from build123d import *

# Parameters (mm, degrees)
SKETCH1_R           = 2.2
BOSS_EXTRUDE1_DEPTH = 22.2504
FILLET1_R           = 10
FILLET2_R           = 2
FILLET3_R           = 4
FILLET4_R           = 1.5
SKETCH2_R           = 2.15
CUT_EXTRUDE1_DEPTH  = 88.351467531


with BuildPart() as part:
    # Sketch1 → Boss-Extrude1 (new body)
    with BuildSketch(Plane(origin=(0, 0, 0), x_dir=(1, 0, 0), z_dir=(0, 1, 0))):
        Polygon((-5, 6.0452), (28.7, 6.0452), (28.7, 57.4548), (-5, 57.4548), (-5, 69.5452), (37.7, 69.5452), (37.7, -6.0452), (-5, -6.0452), align=None)
        with Locations(Location((0, 0, 0), (0, 0, 90))):
            Circle(SKETCH1_R, mode=Mode.SUBTRACT)
        with Locations(Location((12.7, 0, 0), (0, 0, 90))):
            Circle(SKETCH1_R, mode=Mode.SUBTRACT)
        with Locations(Location((12.7, 63.5, 0), (0, 0, 90))):
            Circle(SKETCH1_R, mode=Mode.SUBTRACT)
        with Locations(Location((0, 63.5, 0), (0, 0, 90))):
            Circle(SKETCH1_R, mode=Mode.SUBTRACT)
        with Locations(Location((33.2, 44.45, 0), (0, 0, 90))):
            Circle(SKETCH1_R, mode=Mode.SUBTRACT)
        with Locations(Location((33.2, 19.05, 0), (0, 0, 90))):
            Circle(SKETCH1_R, mode=Mode.SUBTRACT)
    extrude(amount=BOSS_EXTRUDE1_DEPTH)

    # Fillet1
    fillet1_edges = [part.edges().sort_by_distance(p)[0] for p in [
        (37.7, 11.1252, -69.5452),
        (37.7, 11.1252, 6.0452),
    ]]
    fillet(fillet1_edges, radius=FILLET1_R)

    # Fillet2
    fillet2_edges = [part.edges().sort_by_distance(p)[0] for p in [
        (28.7, 11.1252, -6.0452),
        (28.7, 11.1252, -57.4548),
    ]]
    fillet(fillet2_edges, radius=FILLET2_R)

    # Fillet3
    fillet3_edges = [part.edges().sort_by_distance(p)[0] for p in [
        (-5, 11.1252, 6.0452),
        (-5, 11.1252, -6.0452),
        (-5, 11.1252, -57.4548),
        (-5, 11.1252, -69.5452),
    ]]
    fillet(fillet3_edges, radius=FILLET3_R)

    # Fillet4
    fillet4_edges = [part.edges().sort_by_distance(p)[0] for p in [
        (13.35, 0, -69.5452),
        (13.35, 22.2504, -69.5452),
        (37.7, 0, -31.75),
        (34.771067812, 0, 3.116267812),
        (34.771067812, 0, -66.616267812),
        (37.7, 22.2504, -31.75),
        (34.771067812, 22.2504, 3.116267812),
        (34.771067812, 22.2504, -66.616267812),
        (28.7, 0, -31.75),
        (28.7, 22.2504, -31.75),
        (12.85, 0, -57.4548),
        (12.85, 22.2504, -57.4548),
        (28.114213562, 0, -56.869013562),
        (28.114213562, 22.2504, -56.869013562),
        (28.114213562, 0, -6.630986438),
        (28.114213562, 22.2504, -6.630986438),
        (-5, 0, -63.5),
        (-5, 22.2504, -63.5),
        (13.35, 0, 6.0452),
        (-5, 0, 0),
        (12.85, 0, -6.0452),
        (-3.828427125, 0, 4.873627125),
        (-3.828427125, 0, -4.873627125),
        (-3.828427125, 0, -58.626372875),
        (-3.828427125, 0, -68.373627125),
        (12.85, 22.2504, -6.0452),
        (-5, 22.2504, 0),
        (13.35, 22.2504, 6.0452),
        (-3.828427125, 22.2504, 4.873627125),
        (-3.828427125, 22.2504, -4.873627125),
        (-3.828427125, 22.2504, -58.626372875),
        (-3.828427125, 22.2504, -68.373627125),
    ]]
    fillet(fillet4_edges, radius=FILLET4_R)

    # Sketch2 → Cut-Extrude1 (cut, through all)
    with BuildSketch(Plane.XY.offset(6.0452)):
        with Locations((6.35, 11.1252)):
            Circle(SKETCH2_R)
    extrude(amount=-CUT_EXTRUDE1_DEPTH, mode=Mode.SUBTRACT)


solid = part.part
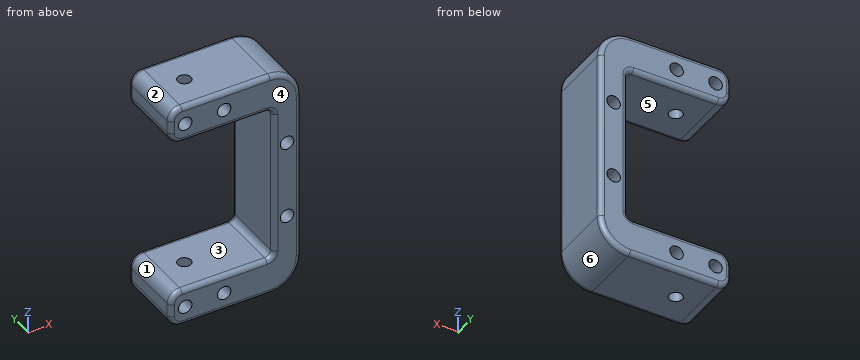
The listing builds one solid part. Answer for the finished solid, in the listing's coordinates (mm). Face numbers are marked on the shaded views. A direction names the side the tool comes from. Round coordinates to 2 decimals unless told otherwise and drop trailing zeros. Loops run counter-clockwise (first coordinate to the right, second up) from the corner with the lowest first, then second, coordinate; pieces in that order, holes last. Notation, with made-up numbers: M 15.5,27.5 L 49.5,27.5 A27 ccw 49.5,54.5 Z; hole C -4,25 d11. An arc over 180 degrees is marked long. Return JSON: item names as keys, results as strings.
Q1. Which of the six approach directions +Z, -Z, +X, -X, +Y, -Y give full straight-line access (tool end or side, diameter ignored) to the marked faces 1 and 2?
Results list:
{"face 1": "-X, +Y, -Y", "face 2": "+Z, -X, +Y, -Y"}
Q2. Find the intervals of material crossed by line 1 along Z through (x, y) = (12.7, 12.25); line 2 along Z through (x, y) = (17.5, 8.25); line 3 along X through (y, z) = (8.5, 0), in increasing order. Write a range as from..to.
Results list:
{"line 1": "z = -69.55..-65.7, -61.3..-57.45, -6.05..-2.2, 2.2..6.05", "line 2": "z = -69.55..-57.45, -6.05..6.05", "line 3": "x = -5..-2.2, 2.2..10.5, 14.9..36.88"}
Q3. Find section A-A, the plane z = -19.05. Determine the outline of the cut face in (x, y), plus the area to 3 significant figures.
Results list:
{"outline": "M 28.7,1.5 A1.5 ccw 30.2,0 L 31,0 L 31,22.25 L 30.2,22.25 A1.5 ccw 28.7,20.75 Z; M 35.4,0 L 36.2,0 A1.5 ccw 37.7,1.5 L 37.7,20.75 A1.5 ccw 36.2,22.25 L 35.4,22.25 Z", "area": "100 mm2"}
Q4. The mould has two halves that part along Z. Classify the marked faces 3, 4, 5 and 6: released by +Z, released by -Z, zero draft, split by the parting line, or undercut.
Results list:
{"face 3": "undercut", "face 4": "zero draft", "face 5": "undercut", "face 6": "released by -Z"}
Q5. Find section B-B, the plane x = 0. Determine the outline of the cut face in (y, z), plus the area to 3 significant figures.
Results list:
{"outline": "M 0,-68.05 A1.5 ccw 1.5,-69.55 L 20.75,-69.55 A1.5 ccw 22.25,-68.05 L 22.25,-65.7 L 0,-65.7 Z; M 0,-61.3 L 22.25,-61.3 L 22.25,-58.95 A1.5 ccw 20.75,-57.45 L 1.5,-57.45 A1.5 ccw 0,-58.95 Z; M 0,-4.55 A1.5 ccw 1.5,-6.05 L 20.75,-6.05 A1.5 ccw 22.25,-4.55 L 22.25,-2.2 L 0,-2.2 Z; M 0,2.2 L 22.25,2.2 L 22.25,4.55 A1.5 ccw 20.75,6.05 L 1.5,6.05 A1.5 ccw 0,4.55 Z", "area": "338 mm2"}
Q6. Find section D-D, the plane z = -32. Determine the outline of the cut face in (x, y), plus the area to 3 significant figures.
Results list:
{"outline": "M 28.7,1.5 A1.5 ccw 30.2,0 L 36.2,0 A1.5 ccw 37.7,1.5 L 37.7,20.75 A1.5 ccw 36.2,22.25 L 30.2,22.25 A1.5 ccw 28.7,20.75 Z", "area": "198 mm2"}
Q7. Find section C-C, the plane x = 25.5. Determine the outline of the cut face in (y, z).
Results list:
{"outline": "M 0,-68.05 A1.5 ccw 1.5,-69.55 L 20.75,-69.55 A1.5 ccw 22.25,-68.05 L 22.25,-58.95 A1.5 ccw 20.75,-57.45 L 1.5,-57.45 A1.5 ccw 0,-58.95 Z; M 0,-4.55 A1.5 ccw 1.5,-6.05 L 20.75,-6.05 A1.5 ccw 22.25,-4.55 L 22.25,4.55 A1.5 ccw 20.75,6.05 L 1.5,6.05 A1.5 ccw 0,4.55 Z"}
Q8. Each of these flat-tipped pins is pushed along its axis until it touches: pin 1 Ø1 at (y, z) = (12, -20.5) entering from -X; pin 2 Ø3.5 at (x, z) = (12.7, 0) entering from -Y; pin 3 Ø1.5 at (y, z) = (14.5, -55.5) entering from -X. Where does it stop, or does it pass through?
Results list:
{"pin 1": "stops at x = 28.7", "pin 2": "passes through", "pin 3": "stops at x = 28.54"}
